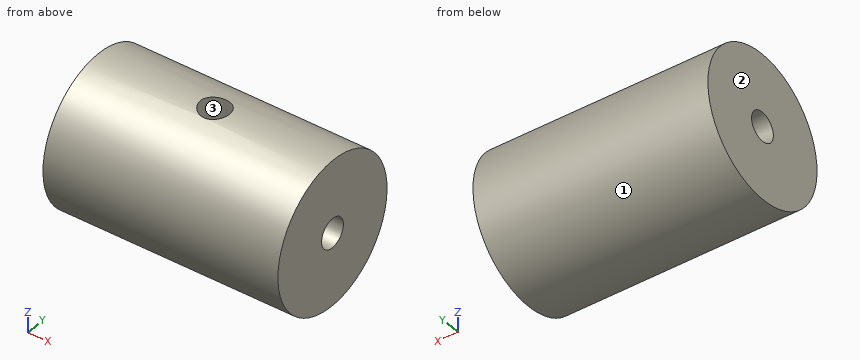
```python
from build123d import *

# Parameters (mm, degrees)
F0_W     = 50.8
F0_H     = 15.875
F2_R     = 3.175
F3_DEPTH = 15.876
F4_R     = 3.175
F5_DEPTH = 50.8010001


# Not quite as in the source:
# - a feature names something its author has since deleted; it is built from what else it names


with BuildPart() as f1:
    # F0 (on Front) → F1 (revolve)
    with BuildSketch(Plane.XZ):
        with Locations((0, 7.9375)):
            Rectangle(F0_W, F0_H)
    revolve(axis=Axis((8.9611150324, 0, 0), (1, 0, 0)))

    # F2 (on Top) → F3 (cut, through all)
    with BuildSketch(Plane.XY):
        Circle(F2_R)
    extrude(amount=F3_DEPTH, mode=Mode.SUBTRACT)

    # F4 (on face) → F5 (cut, through all)
    with BuildSketch(Plane.YZ.offset(25.4)):
        Circle(F4_R)
    extrude(amount=-F5_DEPTH, mode=Mode.SUBTRACT)


solid = f1.part
```
CAD build for the part. Positions are in the model's coordinates, mm. Face numbers are marked on the shaded views. Round coordinates to 2 decimals unless told otherwise and drop trailing zeros. Order: outer loops, then holes, each group sorted by start corner. A loop starts at its lowest first (then second) coordinate and runs counter-clockwise, first axis right, second up. Notation, with made-up numbers: (0.5, -14) - (31.5, -14) arc R14 ccw to (31.5, 9) - close; hole circle Ø5 at (-27.5, 21.25). An arc over 180 degrees is marked (long way). Use CSV: the item, a comma, the result in double quotes. Start each with the question number.
1) Saw through at D-D (y = 13). List the corners of the cut face in (x, z).
2) Saw through at A-A (y = 0). List the corners of the cut face in (x, z) (3 decimals).
3) Saw through at C-C (z = -4). List the corners of the cut face in (x, y), and give its area (3 significant figures).
4) Saw through at B-B (x = -11). List the corners of the cut face in (y, z) (3 decimals), and give its area (3 significant figures).
5) Wall check: L1, parallel to X at y = 0, z = 9.5 (3 decimals); L2, parallel to Z at x = -12, y = 0 (3 decimals). Give the ranges that are in metal, low to high. Write a range as [from, to].
6) Two-plate mould, pull along Y, no slides. Class the marked faces 1, 2 and 3: pulls with the +Y half, pulls with the -Y half, needs draft (parallel to the pull), parting line crosses it, or undercut.
7) Pin check, flat tips, straight feed: pin 1 Ø10 at (x, z) = (-9, -8) entering from +Y; pin 2 Ø12 at (x, z) = (-18.5, 8.5) entering from +Y; pin 3 Ø10 at (x, z) = (7.5, -6) entering from -Y. Stop position of each tip, or through.
Values follow:
1,outline,"(-25.4, -9.11) - (25.4, -9.11) - (25.4, 9.11) - (-25.4, 9.11) - close"
2,outline,"(-25.4, -15.875) - (25.4, -15.875) - (25.4, -3.175) - (-25.4, -3.175) - close; (-25.4, 3.175) - (-3.175, 3.175) - (-3.175, 15.875) - (-25.4, 15.875) - close; (3.175, 3.175) - (25.4, 3.175) - (25.4, 15.875) - (3.175, 15.875) - close"
3,outline,"(-25.4, -15.36) - (25.4, -15.36) - (25.4, 15.36) - (-25.4, 15.36) - close"
3,area,"1,560 mm2"
4,outline,"circle Ø31.75 at (0, 0); hole circle Ø6.35 at (0, 0)"
4,area,"760 mm2"
5,L1,"x = [-25.4, -3.175], [3.175, 25.4]"
5,L2,"z = [-15.875, -3.175], [3.175, 15.875]"
6,face 1,"parting line crosses it"
6,face 2,"needs draft"
6,face 3,"undercut"
7,pin 1,"stops at y = 15.59"
7,pin 2,"stops at y = 15.68"
7,pin 3,"stops at y = -15.84"
